from build123d import *

# Parameters (mm, degrees)
SKETCH1_W           = 50.8
SKETCH1_H           = 3.175
BOSS_EXTRUDE1_DEPTH = 5.08
SKETCH2_R           = 1.27
BOSS_EXTRUDE2_DEPTH = 3.175


with BuildPart() as part:
    # Sketch1 → Boss-Extrude1 (new body)
    with BuildSketch(Plane.XY):
        Rectangle(SKETCH1_W, SKETCH1_H)
    extrude(amount=BOSS_EXTRUDE1_DEPTH)

    # Sketch2 → Boss-Extrude2 (add)
    with BuildSketch(Plane(origin=(0, -1.5875, 0), x_dir=(-1, 0, 0), z_dir=(0, -1, 0))):
        Polygon((-25.4, -5.08), (-38.1, 20.32), (-33.02, 20.32), (-20.32, -5.08), align=None)
        with Locations(Location((-34.29, 17.78, 0), (0, 0, 180))):
            Circle(SKETCH2_R, mode=Mode.SUBTRACT)
    extrude(amount=-BOSS_EXTRUDE2_DEPTH)


solid = part.part
Could you check a few things on this model? Use its own coordinates, in mm. A direction names the side the tool comes from. Coordinates: 2 decimals unless noted, no trailing zeros. Order: outer loops, then holes, each group sorted by start corner. A loop starts at its lowest first (then second) coordinate and runs counter-clockwise, first axis right, second up.
Q1. Suppose I cut it at B-B on y = -0.6. Please give me the cut outline in (x, z), and give its area (3 significant figures).
Q2. Suppose I cut it at D-D on x = 24. Please give me the cut outline in (y, z).
Q3. Suppose I cut it at A-A on x = 34.29. Please give me the cut outline in (y, z), and give its area (3 significant figures).
Q4. Suppose I cut it at C-C on z = -17.78. Please give me the cut outline in (x, y).
Q5. Please list where these lines run through material, in increasing order: L1, parallel to Z at x = -2, y = 0.05; L2, parallel to Z at x = 34.29, y = -0.9; L3, parallel to X at y = 0.7, z = 2.5.
Q6. Will these pins go through, and if not, where does the flat tip stop? pin 1 (1 mm diameter, centred on y = 1, z = -11.5, fed in from +X); pin 2 (3.5 mm diameter, centred on x = 34.29, z = -17.78, fed in from +Y).
Q7. Which directions (+Z, -Z, +X, -X, +Y, -Y) give clear straight access to the entire face, cutting with the end or side of a thin tool? Please do faces 5 (the flat face through (-2, 0, 0)), 6 (the flat face through (9, -1.588, 1)).
Q8. Thinking about a two-plate mould opening in X: for faces 1 (the flat face through (0, 0, 5.08)), 2 (the flat face through (31.66, -0.02, -7.44)), 3 (the flat face through (-25.4, 0, 3)), 4 (the cylindrical face through (34.876, -0.022, -18.907)), which applies, released by +X, released by -X, zero draft, split by the parting line, or undercut?
Answer:
1. outline: (-25.4, 0) - (22.86, 0) - (33.02, -20.32) - (38.1, -20.32) - (25.4, 5.08) - (-25.4, 5.08) - close; hole circle Ø2.54 at (34.29, -17.78)
1. area: 363 mm2
2. outline: (-1.59, -2.28) - (1.59, -2.28) - (1.59, 5.08) - (-1.59, 5.08) - close
3. outline: (-1.59, -20.32) - (1.59, -20.32) - (1.59, -19.05) - (-1.59, -19.05) - close; (-1.59, -16.51) - (1.59, -16.51) - (1.59, -12.7) - (-1.59, -12.7) - close
3. area: 16.1 mm2
4. outline: (31.75, -1.59) - (33.02, -1.59) - (33.02, 1.59) - (31.75, 1.59) - close; (35.56, -1.59) - (36.83, -1.59) - (36.83, 1.59) - (35.56, 1.59) - close
5. L1: z = 0 to 5.08
5. L2: z = -20.32 to -19.05, -16.51 to -12.7
5. L3: x = -25.4 to 26.69
6. pin 1: stops at x = 33.94
6. pin 2: stops at y = 1.59
7. face 5: -Z, -X, +Y, -Y
7. face 6: +Z, -Z, +X, -X, -Y
8. face 1: zero draft
8. face 2: released by +X
8. face 3: released by -X
8. face 4: undercut
